Verification items for the finished model (mm, model axes). A direction names the side the tool comes from. Round coordinates to 2 decimals unless told otherwise and drop trailing zeros. Write each loop counter-clockwise with the first axis right and the second up, starting at its lowest first coordinate (ties: lowest second). Pieces come first, ordered by that corner, then holes. Notation, with made-up numbers: M -27,43 L 18,43 A21 cw 18,57 Z; hole C 63.25,6.5 d11. An arc over 180 degrees is marked long. Use a Markdown table: item, result. Add a question column.
from build123d import *

# Parameters (mm, degrees)
F0_W           = 83.3091139793
F0_H           = 55.9713058174
F1_DEPTH       = 25
F3_D           = 5
F3_DEPTH       = 20
F3_CBORE_D     = 10
F3_CBORE_DEPTH = 5
F3_TIP         = 1.5021515476


with BuildPart() as f1:
    # F0 (on Right) → F1 (new body)
    with BuildSketch(Plane.YZ):
        Rectangle(F0_W, F0_H)
    extrude(amount=F1_DEPTH)

    # F3
    with Locations(Plane.XY.offset(27.9856529087)):
        with Locations((12.5, -27.6769809425), (12.5, -9.8345736042), (12.5, 8.1630079076), (12.5, 23.6527305096)):
            CounterBoreHole(F3_D / 2, F3_CBORE_D / 2, F3_CBORE_DEPTH, depth=F3_DEPTH)
            with Locations((0, 0, -(F3_DEPTH + F3_TIP / 2))):  # 118° drill point
                Cone(0, F3_D / 2, F3_TIP, mode=Mode.SUBTRACT)


solid = f1.part
1. Access from +Z, -Z, +X, -X, +Y, -Y to the whole of each face (thin tool, end or side, straight path). Record for faces 4 (the flat face through (12, 41.655, 0)), 5 (the flat face through (10, -11, 22.986)).
2. Release check for a two-part mould opening along X. For faces 1 (the flat face through (12, -1, 27.986)), 2 (the cylindrical face through (11.42, -32.56, 25.52)), 3 (the flat face through (0, -1, 0)) record: +X half, -X half, draft (parallel to the pull), parting line (faces both ways), or undercut.
3. Cross-section at A-A on z = 14. Enter the section's corners in (x, y), plus the area to 3 significant figures.
4. Depth check by flat-ended pin: pin 1 Ø9 at (x, y) = (12.5, 8.16) entering from +Z; pin 2 Ø10 at (y, z) = (1.5, -14) entering from -X; pin 3 Ø3 at (x, y) = (12, -10.5) entering from +Z. Enter the tip coordinate at first touch or a pass-through.
5. Scan lines: line 1 along Y through (x, z) = (12.5, 26.45); line 2 along Y through (x, z) = (12.5, 18.25); line 3 along Z through (x, y) = (14.25, -12). Record each from-to range of solid material in increasing order. Write a range as from..to.
Answer:
| question | item | result |
|---|---|---|
| 1 | face 4 | +Z, -Z, +X, -X, +Y |
| 1 | face 5 | +Z |
| 2 | face 1 | draft |
| 2 | face 2 | undercut |
| 2 | face 3 | -X half |
| 3 | outline | M 0,-41.65 L 25,-41.65 L 25,41.65 L 0,41.65 Z; hole C 12.5,-27.68 d5; hole C 12.5,-9.83 d5; hole C 12.5,8.16 d5; hole C 12.5,23.65 d5 |
| 3 | area | 2,000 mm^2 |
| 4 | pin 1 | stops at z = 22.99 |
| 4 | pin 2 | stops at x = 0 |
| 4 | pin 3 | stops at z = 7.88 |
| 5 | line 1 | y = -41.65..-32.68, -22.68..-14.83, -4.83..3.16, 13.16..18.65, 28.65..41.65 |
| 5 | line 2 | y = -41.65..-30.18, -25.18..-12.33, -7.33..5.66, 10.66..21.15, 26.15..41.65 |
| 5 | line 3 | z = -27.99..22.99 |
